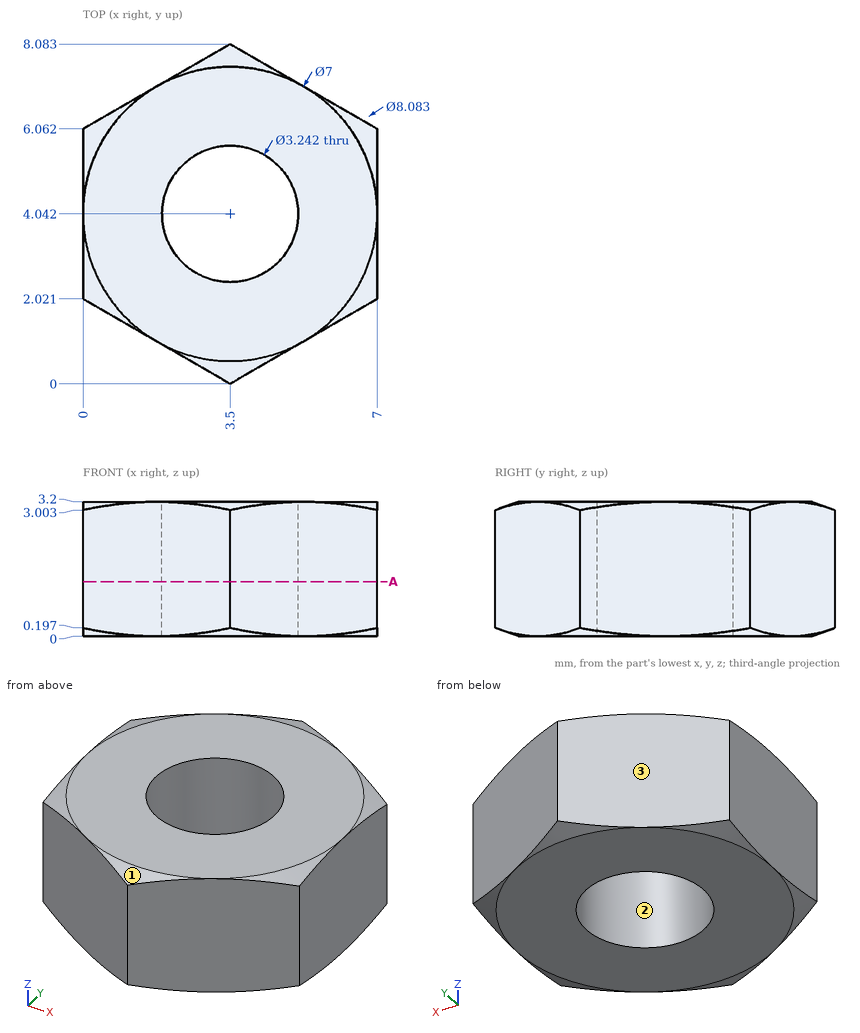
Geometry check sheet. Reference: drawing and pictorial views, mm from the part's lowest x, y, z. Give positions to 0.01 mm unless a question says otherwise; leave off trailing zeros. Write each loop counter-clockwise with the first axis right and the second up, starting at its lowest first coordinate (ties: lowest second). Pieces come first, ordered by that corner, then holes. Notation, with made-up numbers: (76.5, 9.25) - (82.5, 9.25) arc R20 cw to (82.5, 48.25) - close; hole circle Ø11 at (-2.5, -19). An arc over 180 degrees is marked (long way). Use a Markdown table: item, result.
Q1. Section check A-A, the plane z = 1.3. Enter the section's corners in (x, y).
Computed:
| item | result |
|---|---|
| outline | (0, 2.02) - (3.5, 0) - (7, 2.02) - (7, 6.06) - (3.5, 8.08) - (0, 6.06) - close; hole circle Ø3.24 at (3.5, 4.04) |
Q2. Thickness scan on L1, parallel to X at y = 4, z = 1.7; L2, parallel to X at y = 3.5, z = 1.45; L3, parallel to X at y = 1.5, z = 2.25 (1 decimal). Record the ranges inside material, lowest first. Write a range as [from, to].
Computed:
| item | result |
|---|---|
| L1 | x = [0, 1.88], [5.12, 7] |
| L2 | x = [0, 1.97], [5.03, 7] |
| L3 | x = [0.9, 6.1] |
Q3. Draft check along X on the marked faces 1, 2 and 3. Enter one of: pulls with the +X half, pulls with the -X half, needs draft (parallel to the pull), parting line crosses it, or undercut.
Computed:
| item | result |
|---|---|
| face 1 | parting line crosses it |
| face 2 | undercut |
| face 3 | pulls with the -X half |
Q4. Go/stop test with a flat-tipped pin: P1, Ø1.5, axis at y = 1, z = 1.5, coming from the -X side. Record where the tip stops, or that it passes through.
Computed:
| item | result |
|---|---|
| P1 | stops at x = 0.47 |
